The drawing under review shows one solid part. Ordinate dimensions are in mm from its lowest x, y, z. A direction names the side the tool comes from. Coordinates: 2 decimals unless noted, no trailing zeros. Write each loop counter-clockwise with the first axis right and the second up, starting at its lowest first coordinate (ties: lowest second). Pieces come first, ordered by that corner, then holes. Notation, with made-up numbers: (26, 70.25) - (49, 70.25) arc R24 ccw to (49, 96.25) - close; hole circle Ø7 at (70.25, 72). An arc over 180 degrees is marked (long way). Use a Markdown table: item, result.
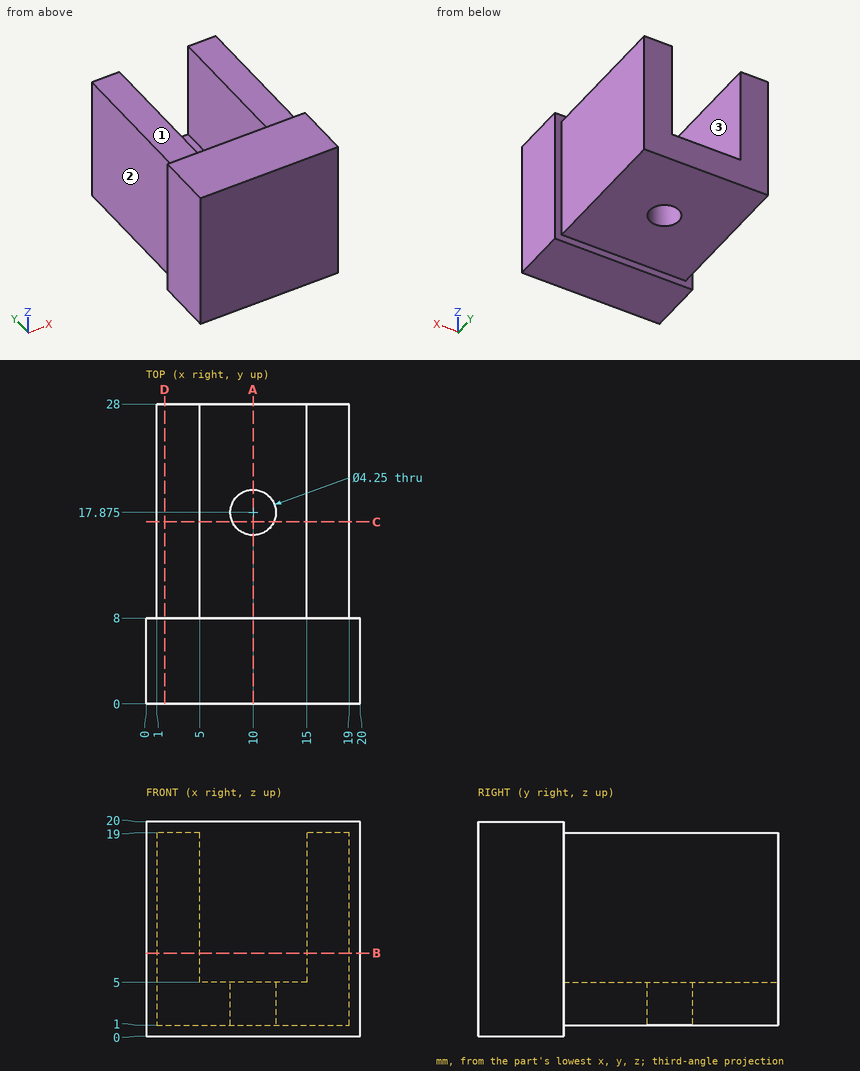
(1) Take a section at D-D on x = 1.75. Write out the cut boundary in (y, z), and give its area (3 significant figures).
Determined:
| item | result |
|---|---|
| outline | (0, 0) - (8, 0) - (8, 1) - (28, 1) - (28, 19) - (8, 19) - (8, 20) - (0, 20) - close |
| area | 520 mm2 |
(2) Machinability: for the marked faces 1, 2 and 3, which of the approach directions +Z, -Z, +X, -X, +Y, -Y give a long, thin tool a straight path to every point of the face, cutting with its end or side? Answer none if there is none.
Determined:
| item | result |
|---|---|
| face 1 | +Z, +X, -X, +Y |
| face 2 | +Z, -Z, -X, +Y |
| face 3 | +Z, +Y |
(3) Take a section at C-C on y = 17. Write out the cut boundary in (x, z).
Determined:
| item | result |
|---|---|
| outline | (1, 1) - (8.06, 1) - (8.06, 5) - (5, 5) - (5, 19) - (1, 19) - close; (11.94, 1) - (19, 1) - (19, 19) - (15, 19) - (15, 5) - (11.94, 5) - close |
(4) Take a section at A-A on x = 10. Write out the cut boundary in (y, z), and give its area (3 significant figures).
Determined:
| item | result |
|---|---|
| outline | (0, 0) - (8, 0) - (8, 1) - (15.75, 1) - (15.75, 5) - (8, 5) - (8, 20) - (0, 20) - close; (20, 1) - (28, 1) - (28, 5) - (20, 5) - close |
| area | 223 mm2 |
(5) Take a section at B-B on z = 7.75. Write out the cut boundary in (x, y).
Determined:
| item | result |
|---|---|
| outline | (0, 0) - (20, 0) - (20, 8) - (19, 8) - (19, 28) - (15, 28) - (15, 8) - (5, 8) - (5, 28) - (1, 28) - (1, 8) - (0, 8) - close |
(6) For L1, parallel to Y at x = 10, z = 1.9; L2, parallel to X at y = 9, z = 8; L3, parallel to Z at x = 7.5, y = 8.5, list the stretches that pass through material, from the lowest coordinate up. Write a range as from..to.
Determined:
| item | result |
|---|---|
| L1 | 0..15.75, 20..28 |
| L2 | 1..5, 15..19 |
| L3 | 1..5 |
(7) For pin 1 (2 mm diameter, centred on x = 17, y = 22, fed in from +Z); pin 2 (3 mm diameter, centred on x = 9.5, y = 21, fed in from +Z); pin 3 (1.5 mm diameter, centred on y = 11, z = 17, fed in from -X); pin 4 (3.5 mm diameter, centred on x = 10, y = 17.875, fed in from -Z), all flat-tipped, find the tip position at first contact; note any pin that passes through.
Determined:
| item | result |
|---|---|
| pin 1 | z = 19 |
| pin 2 | z = 5 |
| pin 3 | x = 1 |
| pin 4 | through |
